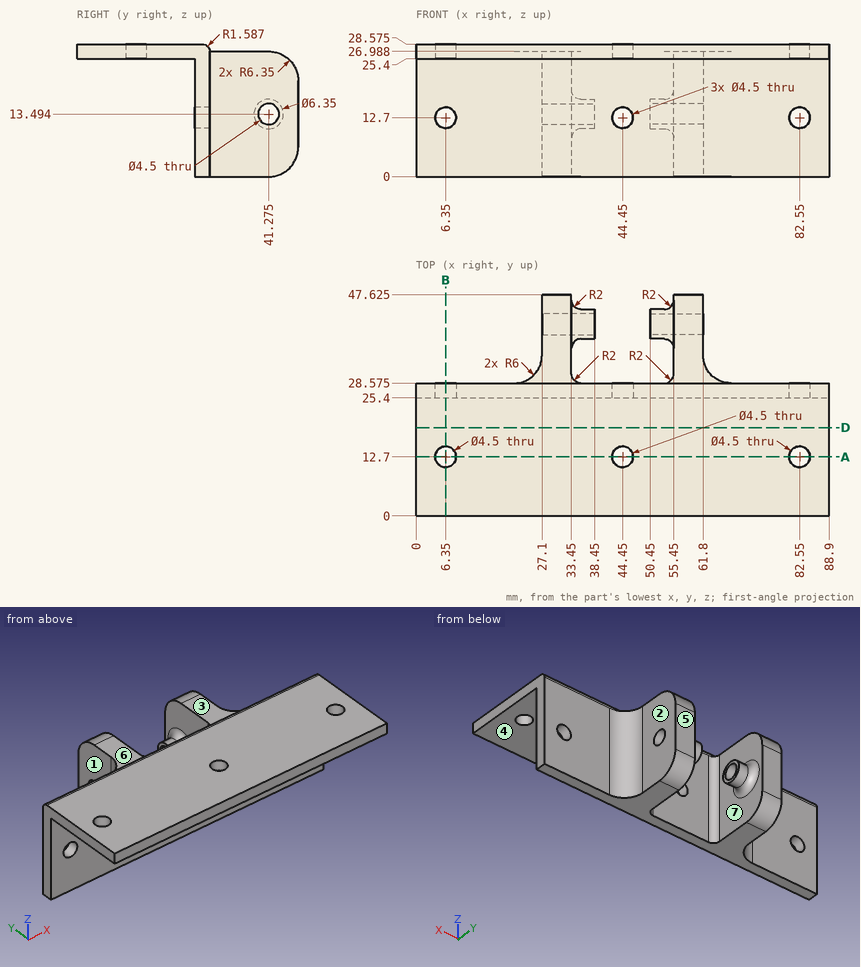
Print and shaded views of the part. All mm, measured from the part's lowest x, y and z. A direction names the side the tool comes from. Round coordinates to 2 decimals unless told otherwise and drop trailing zeros. Write each loop counter-clockwise with the first axis right and the second up, starting at its lowest first coordinate (ties: lowest second). Pieces come first, ordered by that corner, then holes. Notation, with made-up numbers: M 88.25,46 L 122.25,46 A21 cw 122.25,51 Z; hole C 67,37.5 d4. An arc over 180 degrees is marked long. Use a Markdown table: item, result. Add a question column.
1. Slice it at A-A on y = 12.7. Give the cut face in (x, z) (1 decimal).
2. Flat gauge pins, fed straight in: P1, Ø8, axis at x = 52.5, z = 8, coming from the -Y side; P2, Ø5.5, axis at x = 48, z = 7, coming from the +Y side (1 decimal); P3, Ø1.5, axis at x = 49, y = 18, coming from the -Z side; P4, Ø3.5, axis at x = 82.55, y = 12.7, coming from the -Z side. Where does each tip first touch, or does it go through?
3. Slice it at B-B on x = 6.35. Give the number of separate pieces and of enclosed holes in the cut face, then the cut area to 3 significant figures.
4. Drill centre lines: probe 1 along X at (y, z) = (43.5, 3); probe 2 along X at (y, z) = (12.7, 26.2); probe 3 along Y at (x, z) = (61, 13.5) (1 decimal). Where is each one in solid material? Low to high.
5. 3-axis set-ups, long thin cutter, end or side, ignore diameter. For the marked faces 1, 2, 3 and 4: which of +Z, -Z, +X, -X, +Y, -Y reach the whole face in a straight line?
6. Slice it at D-D on y = 19. Give the cut face in (x, z) (1 decimal).
7. Pull direction Y, two halves, no side cores. Call the marked faces 5, 6 and 7: released by +Y, released by -Y, zero draft, split by the parting line, or undercut.
Reply:
| question | item | result |
|---|---|---|
| 1 | outline | M 0,25.4 L 4.1,25.4 L 4.1,28.6 L 0,28.6 Z; M 8.6,25.4 L 42.2,25.4 L 42.2,28.6 L 8.6,28.6 Z; M 46.7,25.4 L 80.3,25.4 L 80.3,28.6 L 46.7,28.6 Z; M 84.8,25.4 L 88.9,25.4 L 88.9,28.6 L 84.8,28.6 Z |
| 2 | P1 | stops at y = 25.4 |
| 2 | P2 | stops at y = 28.6 |
| 2 | P3 | stops at z = 25.4 |
| 2 | P4 | passes through |
| 3 | separate pieces | 3 |
| 3 | enclosed holes | 0 |
| 3 | area | 142 mm^2 |
| 4 | probe 1 | x = 27.1 to 33.45, 55.45 to 61.8 |
| 4 | probe 2 | x = 0 to 4.1, 8.6 to 42.2, 46.7 to 80.3, 84.8 to 88.9 |
| 4 | probe 3 | y = 25.4 to 39, 43.5 to 47.6 |
| 5 | face 1 | +Z, -Z, -X, +Y |
| 5 | face 2 | +Z, -Z, +X, +Y |
| 5 | face 3 | +Z, +X, -X, +Y |
| 5 | face 4 | -Z, +X, -X, -Y |
| 6 | outline | M 0,25.4 L 88.9,25.4 L 88.9,28.6 L 0,28.6 Z |
| 7 | face 5 | released by +Y |
| 7 | face 6 | zero draft |
| 7 | face 7 | undercut |
